Autodesk Inventor part; units mm, degrees
ref_plane "XZ Plane" through (0, 0, 0) normal (0, 1, 0) x (-1, 0, 0)
ref_plane "XY Plane" through (0, 0, 0) normal (0, 0, 1) x (1, 0, 0)
sketch "Sketch1" plane through (0, 0, 0) normal (0, 1, 0) x (-1, 0, 0)
  circle A0 centre (0, 0) radius 12.7
  dimension "d0" = 25.4
extrude "Extrusion1" add sketch "Sketch1" along normal blind 33.7058
sketch "Sketch2" plane through (0, 0, 0) normal (0, -1, 0) x (1, 0, 0)
  circle A0 centre (0, 0) radius 3.175
  dimension "d3" = 6.35
extrude "Extrusion2" cut sketch "Sketch2" against normal blind 21.0058
sketch "Sketch3" plane through (0, 33.7058, 0) normal (0, 1, 0) x (1, 0, 0)
  circle A0 centre (0, 0) radius 6.35
  dimension "d6" = 12.7
extrude "Extrusion3" cut sketch "Sketch3" against normal blind 12.7
ref_plane "Work Plane1" through (3.175, 0, 0) normal (1, 0, 0) x (0, 1, 0)
sketch "Sketch4" plane through (3.175, 0, 0) normal (1, 0, 0) x (0, 1, 0)
  line L0 (0, 0) -> (21.0058, 0) construction
  line L1 (21.0058, -3.175) -> (21.0058, 3.175) construction
  circle A0 centre (10.5029, 0) radius 2.55
  dimension "d10" = 5.1
ref_plane "Work Plane2" through (6.35, 0, 0) normal (1, 0, 0) x (0, 1, 0)
sketch "Sketch5" plane through (6.35, 0, 0) normal (1, 0, 0) x (0, 1, 0)
  line L0 (33.4751, 0) -> (21.0058, 0) construction
  line L1 (21.0058, -3.175) -> (21.0058, 3.175) construction
  circle A0 centre (27.2404, 0) radius 2.55
  point P0 (0, 0)
  dimension "d12" = 5.1
ref_plane "Work Plane3" through (12.7, 0, 0) normal (1, 0, 0) x (0, 1, 0)
sketch "Sketch6" plane through (12.7, 0, 0) normal (1, 0, 0) x (0, 1, 0)
  line L0 (21.0058, -3.175) -> (21.0058, 3.175) construction
  line L1 (21.0058, 0) -> (0, 0) construction
  circle A0 centre (10.5029, 0) radius 2.65
  dimension "d14" = 5.3
sketch "Sketch7" plane through (12.7, 0, 0) normal (1, 0, 0) x (0, 1, 0)
  line L0 (21.0058, -3.175) -> (21.0058, 3.175) construction
  line L1 (21.0058, 0) -> (33.7221, 0) construction
  circle A0 centre (27.364, 0) radius 2.65
  point P0 (0, 0)
  dimension "d15" = 5.3
loft "Loft1" cut profiles "Sketch4", "Sketch6"
loft "Loft2" cut profiles "Sketch5", "Sketch7"
properties part number "Motor Coupler" material "ABS Plastic"
Work out the finished part from the listing and answer in its coordinate system (mm). A direction names the side the tool comes from. Round coordinates to 2 decimals unless told otherwise and drop trailing zeros. Loops run counter-clockwise (first coordinate to the right, second up) from the corner with the lowest first, then second, coordinate; pieces in that order, holes last. Notation, with made-up numbers: M 27,65 L 33,65 A35 cw 33,104 Z; hole C 79.25,2 d2. An arc over 180 degrees is marked long. One line per question, with ' | ' between items. Start each with the question number.
(1) A cutting plane is placed at C-C on x = 4.5. Write down the section's boundary in (y, z), plus the area to 3 significant figures.
(2) For a pull along X with two mould halves and no side action, classify faces 4 (the face through (-0.69, 10.36, -3.1)), 5 (the face through (3.175, 10, -1)), 6 (the face through (-3, 0, -3)), 7 (the face through (-2, 21.006, -3)) as released by +X, released by -X, zero draft, split by the parting line, or undercut.
(3) A cutting plane is placed at B-B on y = 24. Write down the section's boundary in (x, z), plus the area to 3 significant figures.
(4) A cutting plane is placed at D-D on x = -4.5. Write down the section's boundary in (y, z).
(5) A tool of negligible diameter and unlimited length cuts with its end or side. For faces 1 (the face through (8.004, 12.984, 0.781)), 2 (the face through (-3, 33.706, 6)), 3 (the face through (-1.38, 27.44, 6.2)), from which of +Z, -Z, +X, -X, +Y, -Y can it reach the whole face along a straight path? Write none if from no direction.
(6) Flat-ended cylindrical pins translate along their axes: pin 1 Ø2 at (y, z) = (25.5, 7) entering from -X; pin 2 Ø2 at (x, y) = (2.5, 19) entering from -Z; pin 3 Ø3 at (y, z) = (14.5, -3.5) entering from +X. Find the tip coordinate at first contact, or state that the pin passes through.
(7) A cutting plane is placed at A-A on x = 0. Write down the section's boundary in (y, z) (3 decimals), plus the area to 3 significant figures.
(8) Find the intervals of material crossed by line 1 (Z direction, x = 0, y = 6.5) (3 decimals); line 2 (Y direction, x = 6.5, z = 1.5); line 3 (Z direction, x = 0, y = 25), in increasing order.
Geometry check:
1) outline: M 0,-11.88 L 33.71,-11.88 L 33.71,-4.48 L 21.01,-4.48 L 21.01,4.48 L 33.71,4.48 L 33.71,11.88 L 0,11.88 Z; hole C 10.5,0 d5.13 | area: 666 mm²
2) face 4: undercut | face 5: released by +X | face 6: zero draft | face 7: undercut
3) outline: C 0,0 d25.4; hole C 0,0 d12.7 | area: 380 mm²
4) outline: M 0,-11.88 L 33.71,-11.88 L 33.71,-4.48 L 21.01,-4.48 L 21.01,4.48 L 33.71,4.48 L 33.71,11.88 L 0,11.88 Z
5) face 1: +X | face 2: +Z, -Z, +X, -X, +Y | face 3: +Y
6) pin 1: stops at x = -11.19 | pin 2: stops at z = -12.61 | pin 3: stops at x = 12.54
7) outline: M 0,-12.7 L 33.706,-12.7 L 33.706,-6.35 L 21.006,-6.35 L 21.006,-3.175 L 0,-3.175 Z; M 0,3.175 L 21.006,3.175 L 21.006,6.35 L 33.706,6.35 L 33.706,12.7 L 0,12.7 Z | area: 561 mm²
8) line 1: z = -12.7 to -3.175, 3.175 to 12.7 | line 2: y = 0 to 8.4, 12.61 to 25.18, 29.31 to 33.71 | line 3: z = -12.7 to -6.35, 6.35 to 12.7
